Work out the finished part from the listing and answer in its coordinate system (mm). Face numbers are marked on the shaded views. A direction names the side the tool comes from. Give positions to 0.01 mm unless a question says otherwise; leave off trailing zeros. Loops run counter-clockwise (first coordinate to the right, second up) from the corner with the lowest first, then second, coordinate; pieces in that order, holes last. Notation, with made-up numbers: (21, 61) - (67, 61) arc R17 cw to (67, 84) - close; hole circle Ø4 at (-19.5, 76). An arc over 180 degrees is marked (long way). One line per question, with ' | ' between items.
from build123d import *

# Parameters (mm, degrees)
BOSS_EXTRUDE1_DEPTH = 165
SKETCH3_W           = 30
SKETCH3_H           = 32
BOSS_EXTRUDE2_DEPTH = 2
SKETCH4_W           = 30
SKETCH4_H           = 32
BOSS_EXTRUDE3_DEPTH = 2
BOSS_EXTRUDE4_START = 10
BOSS_EXTRUDE4_DEPTH = 10
CUT_EXTRUDE1_DEPTH  = 10
BOSS_EXTRUDE6_DEPTH = 15
CUT_EXTRUDE2_DEPTH  = 15
BOSS_EXTRUDE7_DEPTH = 121
CUT_EXTRUDE3_DEPTH  = 121
SKETCH13_W          = 169
SKETCH13_H          = 30
CUT_EXTRUDE5_DEPTH  = 3
SKETCH14_W          = 169
SKETCH14_H          = 30
BOSS_EXTRUDE8_DEPTH = 3
SKETCH12_W          = 28
SKETCH12_H          = 2
CUT_EXTRUDE6_DEPTH  = 167
SKETCH16_W          = 165
SKETCH16_H          = 26
CUT_EXTRUDE7_DEPTH  = 3


with BuildPart() as part:
    # Sketch2 → Boss-Extrude1 (new body)
    with BuildSketch(Plane(origin=(0, 0, 0), x_dir=(0, 0, -1), z_dir=(1, 0, 0))):
        with BuildLine():
            Line((-13, 0), (-13, 17))
            Line((-13, 17), (-15, 17))
            Line((-15, 17), (-15, -15))
            Line((-15, -15), (15, -15))
            Line((15, -15), (15, 17))
            Line((15, 17), (13, 17))
            Line((13, 17), (13, 0))
            ThreePointArc((13, 0), (0, -13), (-13, 0))
        make_face()
    extrude(amount=BOSS_EXTRUDE1_DEPTH)

    # Sketch3 → Boss-Extrude2 (add)
    with BuildSketch(Plane(origin=(165, 0, 0), x_dir=(0, 0, -1), z_dir=(1, 0, 0))):
        with Locations((0, 1)):
            Rectangle(SKETCH3_W, SKETCH3_H)
    extrude(amount=BOSS_EXTRUDE2_DEPTH)

    # Sketch4 → Boss-Extrude3 (add)
    with BuildSketch(Plane.ZY):
        with Locations((0, 1)):
            Rectangle(SKETCH4_W, SKETCH4_H)
    extrude(amount=BOSS_EXTRUDE3_DEPTH)

    # Sketch5 → Boss-Extrude4 (add)
    with BuildSketch(Plane.ZY.offset(-165).offset(BOSS_EXTRUDE4_START)):
        with BuildLine():
            Line((-13, 17), (-13, 0))
            ThreePointArc((-13, 0), (0, -13), (13, 0))
            Line((13, 0), (13, 17))
            Line((13, 17), (-13, 17))
        make_face()
    extrude(amount=-BOSS_EXTRUDE4_DEPTH)

    # Sketch6 → Cut-Extrude1 (cut)
    with BuildSketch(Plane.ZY.offset(-155)):
        with BuildLine():
            Line((-2, 0), (-2, 17))
            Line((-2, 17), (2, 17))
            Line((2, 17), (2, 0))
            ThreePointArc((2, 0), (0, -2), (-2, 0))
        make_face()
    extrude(amount=-CUT_EXTRUDE1_DEPTH, mode=Mode.SUBTRACT)

    # Sketch8 → Boss-Extrude6 (add)
    with BuildSketch(Plane(origin=(0, 0, 0), x_dir=(0, 0, -1), z_dir=(1, 0, 0))):
        with BuildLine():
            Line((13, 0), (13, 17))
            Line((13, 17), (-13, 17))
            Line((-13, 17), (-13, 0))
            ThreePointArc((-13, 0), (0, -13), (13, 0))
        make_face()
    extrude(amount=BOSS_EXTRUDE6_DEPTH)

    # Sketch9 → Cut-Extrude2 (cut)
    with BuildSketch(Plane(origin=(15, 0, 0), x_dir=(0, 0, -1), z_dir=(1, 0, 0))):
        with BuildLine():
            Line((-2.125, 0), (-2.125, 17))
            Line((-2.125, 17), (2.125, 17))
            Line((2.125, 17), (2.125, 0))
            ThreePointArc((2.125, 0), (0, -2.125), (-2.125, 0))
        make_face()
    extrude(amount=-CUT_EXTRUDE2_DEPTH, mode=Mode.SUBTRACT)

    # Sketch10 → Boss-Extrude7 (add)
    with BuildSketch(Plane(origin=(15, 0, 0), x_dir=(0, 0, -1), z_dir=(1, 0, 0))):
        with BuildLine():
            Line((13, 0), (13, 17))
            Line((13, 17), (-13, 17))
            Line((-13, 17), (-13, 0))
            ThreePointArc((-13, 0), (0, -13), (13, 0))
        make_face()
    extrude(amount=BOSS_EXTRUDE7_DEPTH)

    # Sketch11 → Cut-Extrude3 (cut)
    with BuildSketch(Plane(origin=(136, 0, 0), x_dir=(0, 0, -1), z_dir=(1, 0, 0))):
        with BuildLine():
            Line((-8.5, 0), (-8.5, 17))
            Line((-8.5, 17), (8.5, 17))
            Line((8.5, 17), (8.5, 0))
            ThreePointArc((8.5, 0), (0, -8.5), (-8.5, 0))
        make_face()
    extrude(amount=-CUT_EXTRUDE3_DEPTH, mode=Mode.SUBTRACT)

    # Sketch13 → Cut-Extrude5 (cut)
    with BuildSketch(Plane(origin=(0, 17, 0), x_dir=(1, 0, 0), z_dir=(0, 1, 0))):
        with Locations((82.5, 0)):
            Rectangle(SKETCH13_W, SKETCH13_H)
    extrude(amount=-CUT_EXTRUDE5_DEPTH, mode=Mode.SUBTRACT)

    # Sketch14 → Boss-Extrude8 (add)
    with BuildSketch(Plane(origin=(0, 14, 0), x_dir=(1, 0, 0), z_dir=(0, 1, 0))):
        with Locations((82.5, 0)):
            Rectangle(SKETCH14_W, SKETCH14_H)
    extrude(amount=BOSS_EXTRUDE8_DEPTH)

    # Sketch12 → Cut-Extrude6 (cut)
    with BuildSketch(Plane(origin=(167, 0, 0), x_dir=(0, 0, -1), z_dir=(1, 0, 0))):
        with Locations((0, 15)):
            Rectangle(SKETCH12_W, SKETCH12_H)
    extrude(amount=-CUT_EXTRUDE6_DEPTH, mode=Mode.SUBTRACT)

    # Sketch16 → Cut-Extrude7 (cut)
    with BuildSketch(Plane(origin=(0, 17, 0), x_dir=(1, 0, 0), z_dir=(0, 1, 0))):
        with Locations((82.5, 0)):
            Rectangle(SKETCH16_W, SKETCH16_H)
    extrude(amount=-CUT_EXTRUDE7_DEPTH, mode=Mode.SUBTRACT)


solid = part.part
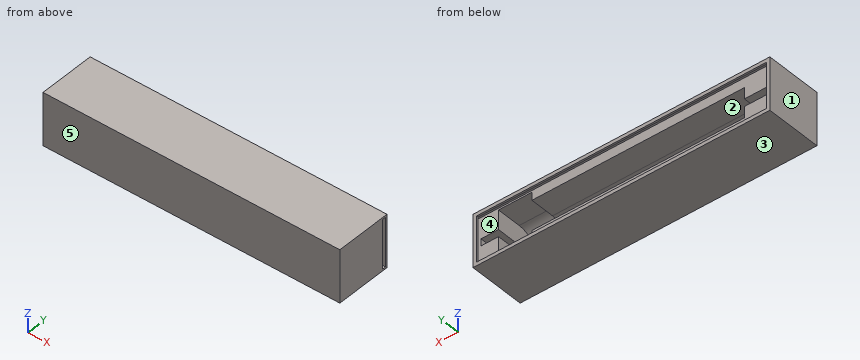
1. Consider L1, parallel to X at y = 0, z = -11; L2, parallel to Z at x = 113.5, y = 7.5; L3, parallel to X at y = 12, z = -5.75. Determine where each line is inside the solid, lowest interval first.
Evaluation:
L1: -2 to 136, 155 to 167 | L2: -15 to -8.5, 8.5 to 15 | L3: -2 to 15, 155 to 167
2. Flat-ended cylindrical pins translate along their axes: pin 1 (1.5 mm diameter, centred on x = 96, z = 2, fed in from +Y); pin 2 (6 mm diameter, centred on x = 98.5, z = -1, fed in from +Y). Find the tip coordinate at first contact, or state that the pin passes through.
Evaluation:
pin 1: y = -8.04 | pin 2: y = -7.5
3. Which of the six approach directions +Z, -Z, +X, -X, +Y, -Y give full straight-line access (tool end or side, diameter ignored) to the marked faces 1 and 2?
Evaluation:
face 1: +Z, -Z, -X, +Y, -Y | face 2: +Y
4. Find section A-A on z = 0. Write down the section's boundary in (x, y) (3 decimals).
Evaluation:
outline: (-2, -15) - (167, -15) - (167, 14) - (165, 14) - (165, -2) - (155, -2) - (155, -13) - (136, -13) - (136, -8.5) - (15, -8.5) - (15, -2.125) - (0, -2.125) - (0, 17) - (-2, 17) - close; (165, 16) - (167, 16) - (167, 17) - (165, 17) - close
5. Find section C-C on y = -6.5. Write down the section's boundary in (x, z).
Evaluation:
outline: (-2, -15) - (167, -15) - (167, 15) - (-2, 15) - close; hole (15, -5.48) - (136, -5.48) - (136, -11.26) - (155, -11.26) - (155, 11.26) - (136, 11.26) - (136, 5.48) - (15, 5.48) - close
6. Find section B-B on x = 34. Write down the section's boundary in (y, z), then the cut area to 3 significant figures.
Evaluation:
outline: (-15, -15) - (17, -15) - (17, -13) - (16, -13) - (16, -14) - (14, -14) - (14, -8.5) - (0, -8.5) arc R8.5 cw to (0, 8.5) - (14, 8.5) - (14, 14) - (16, 14) - (16, 13) - (17, 13) - (17, 15) - (-15, 15) - close | area: 527 mm2
7. Determine the mould class of the marked faces 3, 4 and 5 for opening direction Z: +Z half, -Z half, draft (parallel to the pull), parting line (faces both ways), or undercut.
Evaluation:
face 3: -Z half | face 4: undercut | face 5: draft
